Autodesk Inventor part; units mm, degrees
ref_plane "YZ Plane" through (0, 0, 0) normal (1, 0, 0) x (0, 1, 0)
ref_plane "XZ Plane" through (0, 0, 0) normal (0, 1, 0) x (-1, 0, 0)
ref_plane "XY Plane" through (0, 0, 0) normal (0, 0, 1) x (1, 0, 0)
sketch "Sketch1" plane through (0, 0, 0) normal (0, 0, 1) x (1, 0, 0)
  line L0 (7.62, 0) -> (60.96, 0)
  line L1 (68.58, 7.62) -> (68.58, 35.56)
  line L2 (60.96, 43.18) -> (7.62, 43.18)
  line L3 (0, 35.56) -> (0, 7.62)
  arc A0 (7.62, 43.18) -> (0, 35.56) centre (7.62, 35.56) ccw
  arc A1 (0, 7.62) -> (7.62, 0) centre (7.62, 7.62) ccw
  arc A2 (60.96, 0) -> (68.58, 7.62) centre (60.96, 7.62) ccw
  arc A3 (68.58, 35.56) -> (60.96, 43.18) centre (60.96, 35.56) ccw
  point P0 (0, 0)
  point P1 (68.58, 43.18)
  point P2 (68.58, 0)
  point P3 (0, 43.18)
  dimension "d0" = 68.58
  dimension "d1" = 43.18
  dimension "d2" = 7.62
extrude "Extrusion1" add sketch "Sketch1" along normal blind 25.4
sketch "Sketch2" plane through (0, 0, 25.4) normal (0, 0, 1) x (1, 0, 0)
  line L0 (-0.635, -3.81) -> (69.215, -3.81)
  line L1 (72.39, -0.635) -> (72.39, 43.815)
  line L2 (69.215, 46.99) -> (-0.635, 46.99)
  line L3 (-3.81, 43.815) -> (-3.81, -0.635)
  arc A0 (-0.635, 46.99) -> (-3.81, 43.815) centre (-0.635, 43.815) ccw
  arc A1 (-3.81, -0.635) -> (-0.635, -3.81) centre (-0.635, -0.635) ccw
  arc A2 (69.215, -3.81) -> (72.39, -0.635) centre (69.215, -0.635) ccw
  arc A3 (72.39, 43.815) -> (69.215, 46.99) centre (69.215, 43.815) ccw
  line L4 (60.96, 43.18) -> (7.62, 43.18) construction
  line L5 (0, 35.56) -> (0, 7.62) construction
  point P0 (0, 0)
  point P1 (72.39, 46.99)
  point P2 (72.39, -3.81)
  point P3 (-3.81, 46.99)
  point P4 (34.29, 46.99)
  point P5 (34.29, 43.18)
  point P6 (-3.81, 21.59)
  point P7 (0, 21.59)
  dimension "d5" = 76.2
  dimension "d6" = 50.8
  dimension "d7" = 3.175
extrude "Extrusion2" add sketch "Sketch2" along normal blind 12.7
fillet "Fillet1" radius 3.175 8 edges at (-2.8801, 46.0601, 38.1) (-3.81, 21.59, 38.1) (-2.8801, -2.8801, 38.1) (34.29, -3.81, 38.1) (71.4601, -2.8801, 38.1) (72.39, 21.59, 38.1) (71.4601, 46.0601, 38.1) (34.29, 46.99, 38.1)
sketch "Sketch3" plane through (0, 0, 38.1) normal (0, 0, 1) x (1, 0, 0)
  line L0 (69.215, 46.99) -> (-0.635, 46.99) construction
  line L1 (69.215, 46.99) -> (-0.635, 46.99) construction
  line L2 (-3.81, 43.815) -> (-3.81, -0.635) construction
  line L3 (-3.81, 43.815) -> (-3.81, -0.635) construction
  circle A0 centre (34.29, 21.59) radius 6.75
  circle A1 centre (34.29, 21.59) radius 16 construction
  circle A2 centre (22.9763, 32.9037) radius 2.25
  circle A3 centre (45.6037, 32.9037) radius 2.25
  circle A4 centre (18.29, 21.59) radius 2.25
  circle A5 centre (50.29, 21.59) radius 2.25
  circle A6 centre (22.9763, 10.2763) radius 2.25
  circle A7 centre (45.6037, 10.2763) radius 2.25
  line L4 (22.9763, 32.9037) -> (34.29, 21.59) construction
  line L5 (34.29, 21.59) -> (18.29, 21.59) construction
  point P0 (0, 0)
  point P1 (34.29, 46.99)
  point P2 (-3.81, 21.59)
  point P3 (-3.81, 21.59)
  dimension "d11" = 13.5
  dimension "d14" = 4.5
  dimension "d15" = 32
  dimension "d16" = 45
extrude "Extrusion3" cut sketch "Sketch3" against normal up to surface (38.1 mm away)
chamfer "Chamfer1" distance 1.27 angle 45 6 edges at (43.3537, 32.9037, 0) (20.7263, 32.9037, 0) (16.04, 21.59, 0) (48.04, 21.59, 0) (43.3537, 10.2763, 0) (20.7263, 10.2763, 0)
properties part number "2x3_Spacer_Rear"
For this review, take the finished solid that the model builds, in its own axes (mm). A direction names the side the tool comes from. Coordinates: 2 decimals unless noted, no trailing zeros. Write each loop counter-clockwise with the first axis right and the second up, starting at its lowest first coordinate (ties: lowest second). Pieces come first, ordered by that corner, then holes. Notation, with made-up numbers: (-4, 52.25) - (15, 52.25) arc R27 cw to (15, 84.25) - close; hole circle Ø3 at (52, -29.75). An arc over 180 degrees is marked (long way). Answer in a Markdown table with one row per item. Add a question column.
Q1. Draft analysis for pull direction Y (two halves, no side actions). For faces 5 (the cylindrical face through (-2.9, 46.04, 30.1)), 6 (the cylindrical face through (71.44, 21.9, 37.19)), 7 (the cylindrical face through (25.122, 10.952, 19.943)), 8 (the flat face through (34, -3.81, 30)), state which applies: +Y half, -Y half, draft (parallel to the pull), parting line (faces both ways), or undercut.
Q2. We need section B-B, the plane y = 21.59. State the section outline as (x, z) points (3 decimals).
Q3. We need section A-A, the plane x = 50.29. State the section outline as (y, z) points (3 decimals).
Q4. Tool access review of faces 1 (the flat face through (31, 44, 25.4)), 2 (the flat face through (68.58, 21, 13)), 3 (the cylindrical face through (66.407, 2.291, 12.522)), 4 (the flat face through (34, 0, 13)): name each direction out of +Z, -Z, +X, -X, +Y, -Y from which nothing blocks a thin tool from reaching the whole face with its end or side.
Q5. For probe 1 along X at (y, z) = (21, 33); probe 2 along Y at (x, z) = (50.29, 25); probe 3 along X at (y, z) = (12, 29.5), list the stretches that pass through material, from the lowest coordinate up.
Q6. We need section C-C, the plane y = 27.5. State the section outline as (x, z) points (3 decimals), and give its area (3 significant figures).
Q7. For P1, Ø6, axis at x = 45.6, y = 10.28, coming from the -Z side; P2, Ø12.5, axis at x = 24, z = 14.5, coming from the +Y side; P3, Ø10, axis at y = 19.5, z = 8, coming from the +X side; P4, Ø8, axis at x = 33, y = 37.5, coming from the -Z side, all flat-tipped, find the tip position at first contact; note any pin that passes through.
Q8. We need section D-D, the plane z = 15. State the section outline as (x, y) points.
Answer list:
| question | item | result |
|---|---|---|
| 1 | face 5 | +Y half |
| 1 | face 6 | draft |
| 1 | face 7 | undercut |
| 1 | face 8 | -Y half |
| 2 | outline | (-3.81, 25.4) - (0, 25.4) - (0, 0) - (14.77, 0) - (16.04, 1.27) - (16.04, 38.1) - (-0.635, 38.1) arc R3.175 ccw to (-3.81, 34.925) - close; (20.54, 1.27) - (21.81, 0) - (27.54, 0) - (27.54, 38.1) - (20.54, 38.1) - close; (41.04, 0) - (46.77, 0) - (48.04, 1.27) - (48.04, 38.1) - (41.04, 38.1) - close; (52.54, 1.27) - (53.81, 0) - (68.58, 0) - (68.58, 25.4) - (72.39, 25.4) - (72.39, 34.925) arc R3.175 ccw to (69.215, 38.1) - (52.54, 38.1) - close |
| 3 | outline | (-3.81, 25.4) - (0, 25.4) - (0, 0) - (18.07, 0) - (19.34, 1.27) - (19.34, 38.1) - (-0.635, 38.1) arc R3.175 ccw to (-3.81, 34.925) - close; (23.84, 1.27) - (25.11, 0) - (43.18, 0) - (43.18, 25.4) - (46.99, 25.4) - (46.99, 34.925) arc R3.175 ccw to (43.815, 38.1) - (23.84, 38.1) - close |
| 4 | face 1 | -Z |
| 4 | face 2 | -Z, +X, +Y, -Y |
| 4 | face 3 | -Z, +X, -Y |
| 4 | face 4 | -Z, +X, -X, -Y |
| 5 | probe 1 | x = -3.81 to 16.12, 20.46 to 27.57, 41.01 to 48.12, 52.46 to 72.39 |
| 5 | probe 2 | y = 0 to 19.34, 23.84 to 43.18 |
| 5 | probe 3 | x = -3.81 to 21.53, 24.42 to 44.16, 47.05 to 72.39 |
| 6 | outline | (-3.81, 25.4) - (0, 25.4) - (0, 0) - (31.029, 0) - (31.029, 38.1) - (-0.635, 38.1) arc R3.175 ccw to (-3.81, 34.925) - close; (37.551, 0) - (68.58, 0) - (68.58, 25.4) - (72.39, 25.4) - (72.39, 34.925) arc R3.175 ccw to (69.215, 38.1) - (37.551, 38.1) - close |
| 6 | area | 2,460 mm2 |
| 7 | P1 | stops at z = 0.51 |
| 7 | P2 | stops at y = 43.18 |
| 7 | P3 | stops at x = 68.58 |
| 7 | P4 | stops at z = 0 |
| 8 | outline | (0, 7.62) arc R7.62 ccw to (7.62, 0) - (60.96, 0) arc R7.62 ccw to (68.58, 7.62) - (68.58, 35.56) arc R7.62 ccw to (60.96, 43.18) - (7.62, 43.18) arc R7.62 ccw to (0, 35.56) - close; hole circle Ø4.5 at (18.29, 21.59); hole circle Ø4.5 at (22.98, 10.28); hole circle Ø4.5 at (22.98, 32.9); hole circle Ø13.5 at (34.29, 21.59); hole circle Ø4.5 at (45.6, 10.28); hole circle Ø4.5 at (45.6, 32.9); hole circle Ø4.5 at (50.29, 21.59) |
